```python
from build123d import *

# Parameters (mm, degrees)
SKETCH1_R           = 75
BOSS_EXTRUDE1_DEPTH = 25
SKETCH2_R           = 12
BOSS_EXTRUDE2_DEPTH = 40
BOSS_EXTRUDE3_DEPTH = 3


with BuildPart() as part:
    # Sketch1 → Boss-Extrude1 (new body)
    with BuildSketch(Plane.XY):
        Circle(SKETCH1_R)
    extrude(amount=BOSS_EXTRUDE1_DEPTH)

    # Sketch2 → Boss-Extrude2 (add)
    with BuildSketch(Plane.XY.offset(25)):
        Circle(SKETCH2_R)
    extrude(amount=BOSS_EXTRUDE2_DEPTH)

    # Sketch3 → Boss-Extrude3 (add)
    with BuildSketch(Plane(origin=(0, 0, 0), x_dir=(-1, 0, 0), z_dir=(0, 0, -1))):
        with BuildLine():
            Line((0, 0), (0, 75))
            add(Edge.make_bspline(
                [(7.949037258, 74.577562354), (3.986254227, 74.999822237), (0, 75)],
                knots=[0, 0, 0, 1, 1, 1], degree=2))
            Line((7.949037258, 74.577562354), (7.949037258, 0))
            Line((7.949037258, 0), (0, 0))
        make_face()
    extrude(amount=BOSS_EXTRUDE3_DEPTH)


solid = part.part
```
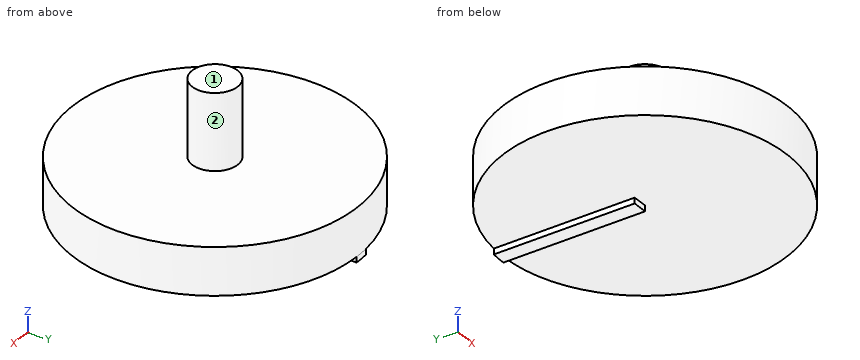
Input: part model. Units: mm. Frame: model coordinates. Face numbers are marked on the shaded views. A direction names the side the tool comes from. Round coordinates to 2 decimals unless told otherwise and drop trailing zeros. Loops run counter-clockwise (first coordinate to the right, second up) from the corner with the lowest first, then second, coordinate; pieces in that order, holes last. Notation, with made-up numbers: (19.25, 70) - (67.25, 70) arc R11 ccw to (67.25, 78) - close; hole circle Ø3 at (-26.75, 29). An arc over 180 degrees is marked (long way). One line per item, written item: value. Start each with the question number.
(1) Contact query for flat-ended pins moving along their axis: P1, Ø10, axis at x = -51.5, y = -39.5, coming from the -Z side; P2, Ø6, axis at y = 11.5, z = 48.5, coming from the -X side; P3, Ø0.9, axis at y = 27.5, z = -1, coming from the +X side. Output: stop coordinate, or through.
(2) Access query for the marked faces 1 and 2. Directions: +Z, -Z, +X, -X, +Y, -Y. A direction counts if a zero-diameter tool reaches every point of the face in a straight line with its end or side. Return the directions, or none.
(3) Ray query, line 1 (Z direction, x = 57, y = 33); line 2 (Y direction, x = -2, z = 33.5); line 3 (Y direction, x = 12, z = 5). Return the intervals inside material, ascending. Write a range as [from, to].
(4) Section A-A, the plane z = 9.5. Return loops of the section in (x, y), plus the area to 3 significant figures.
(5) Section C-C, the plane x = 18. Return loops of the section in (y, z), plus the area to 3 significant figures.
(6) Section B-B, the plane y = 47. Return loops of the section in (x, z).
(7) Section D-D, the plane x = -25. Return loops of the section in (y, z), plus the area to 3 significant figures.
Results below:
1. P1: z = 0
1. P2: x = -8.47
1. P3: x = 0
2. face 1: +Z, +X, -X, +Y, -Y
2. face 2: +Z
3. line 1: [0, 25]
3. line 2: [-11.83, 11.83]
3. line 3: [-74.03, 74.03]
4. outline: circle Ø150 at (0, 0)
4. area: 17,700 mm^2
5. outline: (-72.81, 0) - (72.81, 0) - (72.81, 25) - (-72.81, 25) - close
5. area: 3,640 mm^2
6. outline: (-58.45, 0) - (-7.95, 0) - (-7.95, -3) - (0, -3) - (0, 0) - (58.45, 0) - (58.45, 25) - (-58.45, 25) - close
7. outline: (-70.71, 0) - (70.71, 0) - (70.71, 25) - (-70.71, 25) - close
7. area: 3,540 mm^2
